Part print with two shaded views. Sizes in mm from the minimum x, y, z corner. A direction names the side the tool comes from. Coordinates: 2 decimals unless noted, no trailing zeros. Write each loop counter-clockwise with the first axis right and the second up, starting at its lowest first coordinate (ties: lowest second). Pieces come first, ordered by that corner, then holes. Notation, with made-up numbers: (-25.75, 84.5) -> (0.25, 84.5) arc R14 cw to (0.25, 104.5) -> close; hole circle Ø9 at (60, 35.25). An arc over 180 degrees is marked (long way). Write item = value, one per line. Start each with the question number.
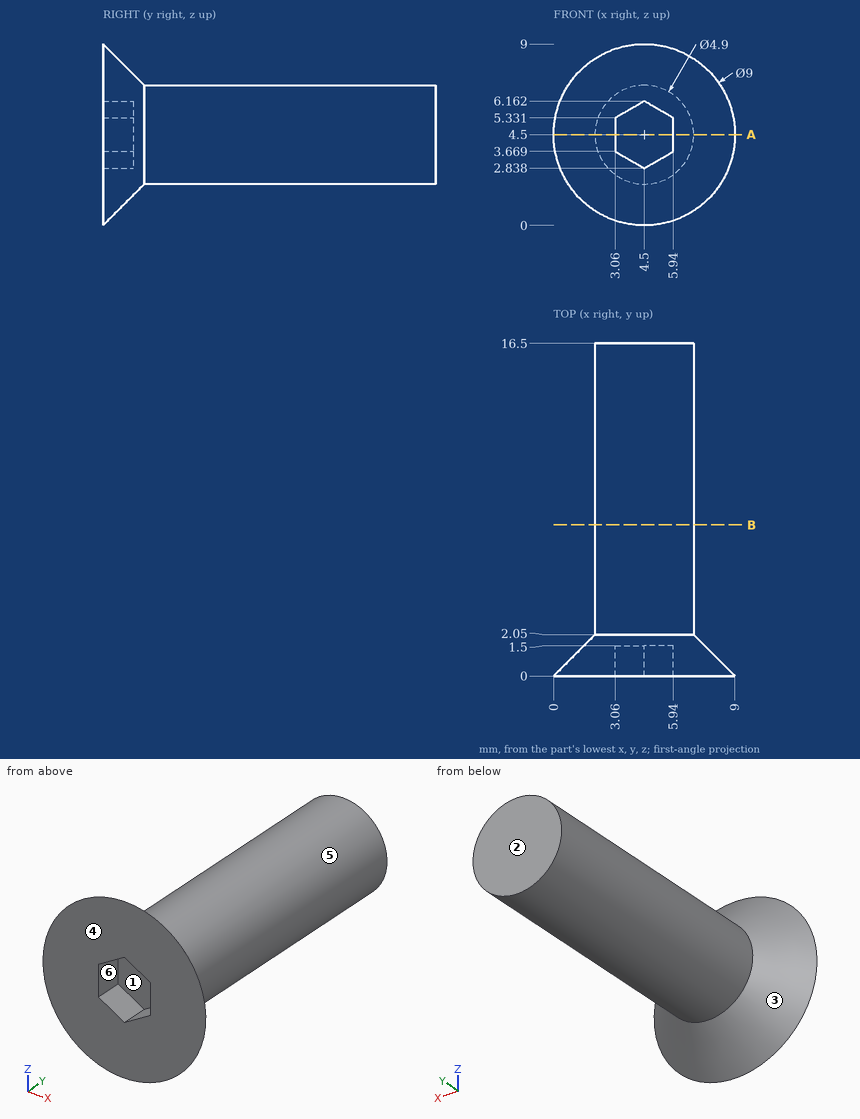
(1) Mould opens along Z. For the marked faces 1, 2 and 3 say: released by +Z, released by -Z, zero draft, split by the parting line, or undercut.
(2) Saw through at A-A (z = 4.5). Give the cut face in (x, y).
(3) 3-axis set-ups, long thin cutter, end or side, ignore diameter. For the marked faces 4, 5 and 6: which of +Z, -Z, +X, -X, +Y, -Y reach the whole face in a straight line?
(4) Drill centre lines: line 1 along X through (y, z) = (1, 2); line 2 along X through (y, z) = (1.25, 3) (1 decimal); line 3 along Y through (x, z) = (1.25, 5.5). Where is each one in solid material? Low to high.
(5) Saw through at B-B (y = 7.5). Give the cut face in (x, z).
(6) Drop flat-ended pins along their axis: pin 1 Ø4 at (x, y) = (8, 11.5) entering from +Z; pin 2 Ø1.4 at (x, z) = (4, 4) entering from -Y; pin 3 Ø1.6 at (y, z) = (1, 4.5) entering from +X. Give the stop position or say it passes through.
Returned:
q1.face_1 = undercut
q1.face_2 = zero draft
q1.face_3 = split by the parting line
q2.outline = (0, 0) -> (3.06, 0) -> (3.06, 1.5) -> (5.94, 1.5) -> (5.94, 0) -> (9, 0) -> (6.95, 2.05) -> (6.95, 16.5) -> (2.05, 16.5) -> (2.05, 2.05) -> close
q3.face_4 = +Z, -Z, +X, -X, -Y
q3.face_5 = +Y
q3.face_6 = -Y
q4.line_1 = 2.05 to 6.95
q4.line_2 = 1.6 to 4.2, 4.8 to 7.4
q4.line_3 = 0 to 1.1
q5.outline = circle Ø4.9 at (4.5, 4.5)
q6.pin_1 = 6.44
q6.pin_2 = 1.5
q6.pin_3 = 8.8
